Autodesk Inventor part; units mm, degrees
ref_plane "YZ Plane" through (0, 0, 0) normal (1, 0, 0) x (0, 1, 0)
ref_plane "XZ Plane" through (0, 0, 0) normal (0, 1, 0) x (-1, 0, 0)
ref_plane "XY Plane" through (0, 0, 0) normal (0, 0, 1) x (1, 0, 0)
sketch "Sketch1" plane through (0, 0, 0) normal (0, 0, 1) x (1, 0, 0)
  line L0 (0, 0) -> (-40, 0)
  line L1 (-40, 0) -> (-40, 15)
  line L2 (-40, 15) -> (0, 15)
  line L3 (0, 15) -> (0, 0)
  line L4 (1, -1) -> (-41, -1)
  line L5 (-41, -1) -> (-41, 16)
  line L6 (-41, 16) -> (1, 16)
  line L7 (1, 16) -> (1, -1)
  circle A0 centre (-1.293, 13.707) radius 0.75
  circle A1 centre (-1.293, 1.293) radius 0.75
  circle A2 centre (-38.707, 1.293) radius 0.75
  circle A3 centre (-38.707, 13.707) radius 0.75
  circle A4 centre (-38.707, 13.707) radius 1.293
  circle A5 centre (-38.707, 1.293) radius 1.293
  circle A6 centre (-1.293, 1.293) radius 1.293
  circle A7 centre (-1.293, 13.707) radius 1.293
  dimension "d0" = 40
  dimension "d1" = 15
  dimension "d2" = 42
  dimension "d3" = 17
  dimension "d4" = 1
  dimension "d6" = 1
  dimension "d7" = 1
  dimension "d8" = 1.5
  dimension "d9" = 1.5
  dimension "d10" = 1.293
  dimension "d11" = 1.293
  dimension "d12" = 1.293
  dimension "d13" = 1.293
  dimension "d14" = 1.5
  dimension "d15" = 1.293
  dimension "d16" = 1.293
  dimension "d17" = 1.5
  dimension "d18" = 1.293
  dimension "d19" = 1.293
extrude "Extrusion1" add sketch "Sketch1" along normal blind 6 contours L4 L5 L6 L7
extrude "Extrusion2" add sketch "Sketch1" along normal blind 1 contours L0 A6 L3 | L0 A5 L1 A4 L2 A7 L3 A6 | A6 | L0 L1 A5 | A5 | A7 L2 L3 | A7 | L1 L2 A4 | A4 | A0 | A1 | A2 | A3
extrude "Extrusion4" add sketch "Sketch1" along normal blind 5 contours A6 | A5 | A7 | A4
thread "Thread1"
thread "Thread2"
thread "Thread3"
thread "Thread4"
fillet "Fillet1" radius 1 8 edges at (1, 16, 3) (-41, 16, 3) (-41, -1, 3) (1, -1, 3) (1, 7.5, 0) (-20, 16, 0) (-20, -1, 0) (-41, 7.5, 0)
properties part number "Bottom part of case"
Input: part model. Units: mm. Frame: model coordinates. A direction names the side the tool comes from. Coordinates: 2 decimals unless noted, no trailing zeros. Write each loop counter-clockwise with the first axis right and the second up, starting at its lowest first coordinate (ties: lowest second). Pieces come first, ordered by that corner, then holes. Notation, with made-up numbers: (-24, 61.25) -> (8, 61.25) arc R31 ccw to (8, 99.25) -> close; hole circle Ø6 at (39.5, -7.5). An arc over 180 degrees is marked (long way). Answer as a JSON object with one key per item and string values.
1. Access query for faces 4 (the face through (-37.99, 1.07, 2.97)), 5 (the face through (-20, 16, 3)). Directions: +Z, -Z, +X, -X, +Y, -Y. A direction counts if a zero-diameter tool reaches every point of the face in a straight line with its end or side. Return the directions, or none.
Result set:
{"face 4": "+Z", "face 5": "+Z, -Z, +X, -X, +Y"}
2. First-contact query: P1, Ø4, axis at x = -17.5, y = 9, coming from the +Z side; P2, Ø0.6, axis at x = -39.5, y = 0.5, coming from the +Z side. Flat tips, straight axial feed; report the tip coordinate or a pass-through.
Result set:
{"P1": "stops at z = 1", "P2": "stops at z = 5"}
3. Section B-B on y = 4.5. Return the cut outline in (x, z).
Result set:
{"outline": "(-41, 1) arc R1 ccw to (-40, 0) -> (0, 0) arc R1 ccw to (1, 1) -> (1, 6) -> (0, 6) -> (0, 1) -> (-40, 1) -> (-40, 6) -> (-41, 6) -> close"}
4. Material intervals for line 1 (Y direction, x = -37, z = 2.3); line 2 (X direction, y = 4.25, z = 3.2); line 3 (Z direction, x = -15, y = 5), sorted ascending. Write a range as from..to.
Result set:
{"line 1": "y = -1..0, 15..16", "line 2": "x = -41..-40, 0..1", "line 3": "z = 0..1"}
5. Section C-C on x = -8.5. Return the cut outline in (y, z), then the cut area to 3 significant figures.
Result set:
{"outline": "(-1, 1) arc R1 ccw to (0, 0) -> (15, 0) arc R1 ccw to (16, 1) -> (16, 6) -> (15, 6) -> (15, 1) -> (0, 1) -> (0, 6) -> (-1, 6) -> close", "area": "26.6 mm2"}
6. Section A-A on z = 4.3. Count the separate pieces of the cut face and the enclosed holes in it, then the cut area to 3 significant figures.
Result set:
{"separate pieces": "5", "enclosed holes": "5", "area": "127 mm2"}
7. Mould query, pull axis X, two halves, no side actions, for faces 1 (the face through (-1, 14, 1)), 2 (the face through (-40.715, -0.699, 3.535)), 3 (the face through (-20.1, -0.6, 6)). Classes: released by +X, released by -X, zero draft, split by the parting line, or undercut.
Result set:
{"face 1": "undercut", "face 2": "released by -X", "face 3": "zero draft"}
